```python
from build123d import *

# Parameters (mm, degrees)
ESQUISSE1_W             = 50
ESQUISSE1_H             = 130
EXTRUSION1_DEPTH        = 6
ESQUISSE3_R             = 2.6
ESQUISSE3_R_2           = 1.6
ENL_V_MAT_EXTRU_1_DEPTH = 6
ENL_V_MAT_EXTRU_2_DEPTH = 20
CONG_1_R                = 10
CONG_2_R                = 5


with BuildPart() as part:
    # Esquisse1 → Extrusion1 (new body)
    with BuildSketch(Plane.XY):
        with Locations((-2.937764085, -11.025)):
            Rectangle(ESQUISSE1_W, ESQUISSE1_H)
    extrude(amount=EXTRUSION1_DEPTH)

    # Esquisse3 → Enlèv. mat.-Extru.1 (cut)
    with BuildSketch(Plane.XY.offset(6)):
        with Locations((-21.937764085, 47.975)):
            Circle(ESQUISSE3_R)
        with Locations((16.062235915, -6.025)):
            Circle(ESQUISSE3_R_2)
        Polygon((-7.937764085, 53.975), (22.062235915, 3.975), (22.062235915, 53.975), align=None)
    extrude(amount=-ENL_V_MAT_EXTRU_1_DEPTH, mode=Mode.SUBTRACT)

    # Esquisse4 → Enlèv. mat.-Extru.2 (cut)
    with BuildSketch(Plane.XY.offset(6)):
        with BuildLine():
            Line((-27.937764085, 36.785641628), (-27.937764085, -63.408020344))
            ThreePointArc((-27.937764085, -63.408020344), (0.051382603, -13.311189358), (-27.937764085, 36.785641628))
        make_face()
        with BuildLine():
            Line((-17.937764085, 53.975), (9.122584116, 53.975))
            Line((9.122584116, 53.975), (35.098718701, 7.628755869))
            Line((35.098718701, 7.628755869), (22.062235915, -70.564710485))
            ThreePointArc((22.062235915, -70.564710485), (8.455247334, -43.39579421), (22.062235915, -16.226877934))
            ThreePointArc((22.062235915, -16.226877934), (9.650339, 23.197650833), (-17.937764085, 53.975))
        make_face()
    extrude(amount=-ENL_V_MAT_EXTRU_2_DEPTH, mode=Mode.SUBTRACT)

    # Congé1
    cong_1_edges = [part.edges().sort_by_distance(p)[0] for p in [
        (-27.937764085, 36.785641628, 3),
        (-27.937764085, -63.408020344, 3),
        (22.062235915, -16.226877934, 3),
    ]]
    fillet(cong_1_edges, radius=CONG_1_R)

    # Congé2
    cong_2_edges = [part.edges().sort_by_distance(p)[0] for p in [
        (22.062235915, -70.564710485, 3),
        (-17.937764085, 53.975, 3),
        (-27.937764085, 53.975, 3),
    ]]
    fillet(cong_2_edges, radius=CONG_2_R)


solid = part.part
```
The model under review builds one solid part; all positions refer to its coordinate system, in mm. A direction names the side the tool comes from. Coordinates: 2 decimals unless noted, no trailing zeros. Order: outer loops, then holes, each group sorted by start corner. A loop starts at its lowest first (then second) coordinate and runs counter-clockwise, first axis right, second up. Notation, with made-up numbers: (31, -21.5) -> (54, -21.5) arc R27 ccw to (54, 16.5) -> close; hole circle Ø2 at (65.25, 18.25). An arc over 180 degrees is marked (long way). Answer in a Markdown table with one row per item. Add a question column.
Item 1: Machinability: for faces 5 (the cylindrical face through (-26.83, 37.52, 2.96)), 6 (the flat face through (-3, -76.025, 3)), 7 (the cylindrical face through (21.617, -70.9, 2.958)), which of the approach directions +Z, -Z, +X, -X, +Y, -Y give a long, thin tool a straight path to every point of the face, cutting with its end or side? Answer none if there is none.
Item 2: We need section D-D on x = 12. Write out the cut boundary in (y, z) (3 decimals).
Item 3: To check wall thickness, follow probe 1 along Y at (x, z) = (-23.5, 5.75) (3 decimals); probe 2 along Y at (x, z) = (-22, 3.25) (3 decimals); probe 3 along Y at (x, z) = (12, 5.5) (3 decimals). State the ranges of each line that lie inside material, in increasing order.
Item 4: Mouldability with a two-part tool opening along X and no side actions: class faces 1 (the cylindrical face through (8.937, 24.429, 3.042)), 2 (the flat face through (2, -25, 0)), 3 (the cylindrical face through (14.464, -5.955, 3.042)), 4 (the cylindrical face through (-20.54, 50.167, 3.042)) as +X half, -X half, draft (parallel to the pull), parting line (faces both ways), or undercut.
Item 5: Clearance check with flat-ended pins moving along their axes: pin 1 (3 mm diameter, centred on y = -38, z = 4, fed in from +X); pin 2 (8.5 mm diameter, centred on x = -21.94, y = 47.98, fed in from -Z); pin 3 (3 mm diameter, centred on y = -13, z = 4, fed in from +X); pin 4 (2 mm diameter, centred on y = 3.5, z = 2, fed in from -X). State where each tip first meets the part, or that it passes through.
Item 6: We need section A-A on x = -2. Write out the cut boundary in (y, z) (3 decimals), plus the area to 3 significant figures.
Item 7: We need section C-C on y = -59.5. Write out the cut boundary in (x, z), plus the area to 3 significant figures.
Item 8: We need section B-B on z = 1.75. Give the number of separate pieces and of enclosed holes in the cut face, plus the area to 3 significant figures.
Final values:
| question | item | result |
|---|---|---|
| 1 | face 5 | +Z, -Z, -X |
| 1 | face 6 | +Z, -Z, +X, -X, -Y |
| 1 | face 7 | +Z, -Z, +X |
| 2 | outline | (-76.025, 0) -> (-58.494, 0) -> (-58.494, 6) -> (-76.025, 6) -> close; (-28.297, 0) -> (18.819, 0) -> (18.819, 6) -> (-28.297, 6) -> close |
| 3 | probe 1 | y = -76.025 to -60.389, 33.766 to 45.897, 50.053 to 53.943 |
| 3 | probe 2 | y = -76.025 to -59.226, 32.604 to 45.376, 50.574 to 53.975 |
| 3 | probe 3 | y = -76.025 to -58.494, -28.297 to 18.819 |
| 4 | face 1 | +X half |
| 4 | face 2 | draft |
| 4 | face 3 | undercut |
| 4 | face 4 | undercut |
| 5 | pin 1 | stops at x = 9.16 |
| 5 | pin 2 | stops at z = 0 |
| 5 | pin 3 | stops at x = 21.5 |
| 5 | pin 4 | stops at x = -2.71 |
| 6 | outline | (-76.025, 0) -> (-28.711, 0) -> (-28.711, 6) -> (-76.025, 6) -> close; (2.088, 0) -> (39.499, 0) -> (39.499, 6) -> (2.088, 6) -> close |
| 6 | area | 508 mm2 |
| 7 | outline | (-22.34, 0) -> (12.52, 0) -> (12.52, 6) -> (-22.34, 6) -> close |
| 7 | area | 209 mm2 |
| 8 | separate pieces | 1 |
| 8 | enclosed holes | 2 |
| 8 | area | 3,020 mm2 |
